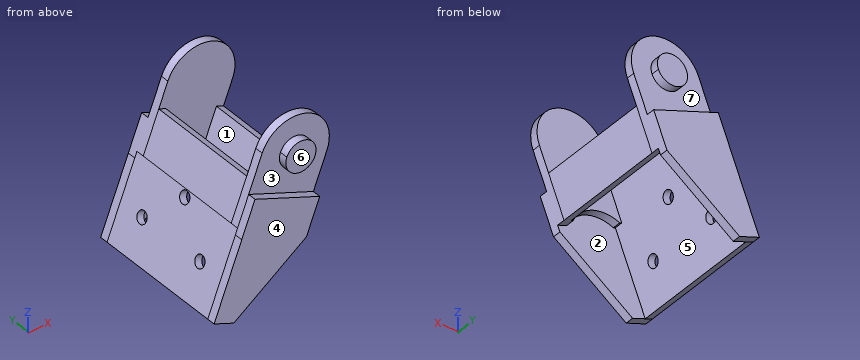
```python
from build123d import *

# Parameters (mm, degrees)
SALIENTE_EXTRUIR1_START   = -2.75
SALIENTE_EXTRUIR1_DEPTH   = 5.5
SALIENTE_EXTRUIR1_2_DEPTH = 2.75
SALIENTE_EXTRUIR2_DEPTH   = 38
SALIENTE_EXTRUIR3_START   = 2.75
SALIENTE_EXTRUIR3_DEPTH   = 2.75
CROQUIS4_W                = 23
CROQUIS4_H                = 43.5
CORTAR_EXTRUIR1_DEPTH     = 8.25
CORTAR_EXTRUIR2_DEPTH     = 2.75
CROQUIS6_W                = 38
CROQUIS6_H                = 22.249999999
CORTAR_EXTRUIR3_DEPTH     = 16.59246817
CROQUIS7_W                = 3.203765914
CROQUIS7_H                = 38
CORTAR_EXTRUIR4_DEPTH     = 8.25
CROQUIS8_W                = 3.203765916
CROQUIS8_H                = 38
CORTAR_EXTRUIR5_DEPTH     = 8.25
CROQUIS9_W                = 14
CROQUIS9_H                = 38
CORTAR_EXTRUIR6_DEPTH     = 0.703765915
CROQUIS10_W               = 14
CROQUIS10_H               = 38
CORTAR_EXTRUIR7_DEPTH     = 0.703765915
SALIENTE_EXTRUIR4_START   = 2.75
SALIENTE_EXTRUIR4_DEPTH   = 2.75
CORTAR_EXTRUIR8_DEPTH     = 2.75
CROQUIS13_W               = 12.249999999
CROQUIS13_H               = 2.75
CORTAR_EXTRUIR9_DEPTH     = 74.034358614
CROQUIS14_W               = 12.249999999
CROQUIS14_H               = 2.75
CORTAR_EXTRUIR10_DEPTH    = 74.034358614
CROQUIS15_W               = 5
CROQUIS15_H               = 2.75
CROQUIS16_W               = 5
CROQUIS16_H               = 2.75
TALADRO1_D                = 10.15
TALADRO1_DEPTH            = 2.75
TALADRO2_D                = 10.15
CORTAR_EXTRUIR11_DEPTH    = 2.75
CORTAR_EXTRUIR12_START    = -2.75
CORTAR_EXTRUIR12_DEPTH    = 2.75
CORTAR_EXTRUIR13_REACH    = 202.135
SALIENTE_EXTRUIR5_DEPTH   = 2.75
SALIENTE_EXTRUIR6_DEPTH   = 2.75
CROQUIS26_W               = 27
CROQUIS26_H               = 43.5
SALIENTE_EXTRUIR7_DEPTH   = 2.5
CROQUIS27_R               = 2
CORTAR_EXTRUIR14_DEPTH    = 2.5


with BuildPart() as part:
    # Saliente-Extruir1: read off the stored shape, not the designer's step
    # Saliente-Extruir1 outline → Saliente-Extruir1 (new body)
    with BuildSketch(Plane(origin=(0, 40.75, 0), x_dir=(-1, 0, 0), z_dir=(0, 1, 0)).offset(SALIENTE_EXTRUIR1_START)):
        with BuildLine():
            Line((161.177139208, 19.345694485), (182.584423689, 27.755698719))
            Line((182.584423689, 27.755698719), (171.432026769, 56.143619441))
            ThreePointArc((171.432026769, 56.143619441), (156.523382412, 62.642259564), (150.024742289, 47.733615207))
            Line((150.024742289, 47.733615207), (161.177139208, 19.345694485))
        make_face()
    extrude(amount=SALIENTE_EXTRUIR1_DEPTH)

    # Saliente-Extruir1 2 outline → Saliente-Extruir1 2 (add)
    with BuildSketch(Plane(origin=(0, 40.75, 0), x_dir=(-1, 0, 0), z_dir=(0, 1, 0))):
        with BuildLine():
            ThreePointArc((161.177139208, 19.345694485), (176.085783565, 12.847054362), (182.584423687, 27.755698719))
            Line((182.584423687, 27.755698719), (161.177139208, 19.345694485))
        make_face()
    extrude(amount=SALIENTE_EXTRUIR1_2_DEPTH)

    # Croquis2 → Saliente-Extruir2 (add)
    with BuildSketch(Plane.XZ.offset(-38)):
        Polygon((-171.432026768, 56.143619442), (-150.024742288, 47.733615205), (-161.177139209, 19.345694483), (-182.584423689, 27.755698719), align=None)
    extrude(amount=SALIENTE_EXTRUIR2_DEPTH)

    # Croquis3 → Saliente-Extruir3 (add)
    with BuildSketch(Plane.XZ.offset(SALIENTE_EXTRUIR3_START)):
        with BuildLine():
            Line((-182.584423688, 27.755698719), (-171.432026768, 56.143619441))
            ThreePointArc((-171.432026768, 56.143619441), (-156.523382412, 62.642259564), (-150.024742289, 47.733615207))
            Line((-150.024742289, 47.733615207), (-161.177139208, 19.345694485))
            Line((-161.177139208, 19.345694485), (-182.584423688, 27.755698719))
        make_face()
    extrude(amount=-SALIENTE_EXTRUIR3_DEPTH)

    # Croquis4 → Cortar-Extruir1 (cut)
    with BuildSketch(Plane(origin=(-14.965700114, 0, -38.094511116), x_dir=(-0.9307514991056489, 0, 0.3656523580022251), z_dir=(-0.3656523580022251, 0, -0.9307514991056489))):
        with Locations((168.589662745, 19)):
            Rectangle(CROQUIS4_W, CROQUIS4_H)
    extrude(amount=-CORTAR_EXTRUIR1_DEPTH, mode=Mode.SUBTRACT)

    # Croquis5 → Cortar-Extruir2 (cut)
    with BuildSketch(Plane(origin=(0, 40.75, 0), x_dir=(1, 0, 0), z_dir=(0, 1, 0))):
        with BuildLine():
            Line((-161.142417183, -28.195858914), (-176.585881806, -34.262934025))
            ThreePointArc((-176.585881806, -34.262934025), (-167.602648859, -34.440489141), (-161.142417183, -28.195858914))
        make_face()
    extrude(amount=-CORTAR_EXTRUIR2_DEPTH, mode=Mode.SUBTRACT)

    # Croquis6 → Cortar-Extruir3 (cut)
    with BuildSketch(Plane(origin=(-149.193349022, 0, 58.611670162), x_dir=(0, 1, 0), z_dir=(0.9307514991056486, 0, -0.3656523580022258))):
        with Locations((19, -21.553766865)):
            Rectangle(CROQUIS6_W, CROQUIS6_H)
    extrude(amount=-CORTAR_EXTRUIR3_DEPTH, mode=Mode.SUBTRACT)

    # Croquis7 → Cortar-Extruir4 (cut)
    with BuildSketch(Plane(origin=(-3.8133032, 0, -9.706590403), x_dir=(0.9307514990825102, 0, -0.36565235806112356), z_dir=(0.36565235806112356, 0, 0.9307514990825102))):
        with Locations((-158.691545702, 19)):
            Rectangle(CROQUIS7_W, CROQUIS7_H)
    extrude(amount=-CORTAR_EXTRUIR4_DEPTH, mode=Mode.SUBTRACT)

    # Croquis8 → Cortar-Extruir5 (cut)
    with BuildSketch(Plane(origin=(-3.8133032, 0, -9.706590403), x_dir=(0.9307514990825102, 0, -0.36565235806112356), z_dir=(0.36565235806112356, 0, 0.9307514990825102))):
        with Locations((-178.487779787, 19)):
            Rectangle(CROQUIS8_W, CROQUIS8_H)
    extrude(amount=-CORTAR_EXTRUIR5_DEPTH, mode=Mode.SUBTRACT)

    # Croquis9 → Cortar-Extruir6 (cut)
    with BuildSketch(Plane(origin=(-164.636813645, 0, 64.678745273), x_dir=(-0.3656523580022247, 0, -0.930751499105649), z_dir=(0.930751499105649, 1.4355340193330324e-15, -0.3656523580022247))):
        with Locations((25.678766864, 19)):
            Rectangle(CROQUIS9_W, CROQUIS9_H)
    extrude(amount=-CORTAR_EXTRUIR6_DEPTH, mode=Mode.SUBTRACT)

    # Croquis10 → Cortar-Extruir7 (cut)
    with BuildSketch(Plane(origin=(-149.193349022, 0, 58.611670162), x_dir=(0.3656523580022248, 0, 0.930751499105649), z_dir=(-0.930751499105649, -1.4355340193330322e-15, 0.3656523580022248))):
        with Locations((-25.678766864, 19)):
            Rectangle(CROQUIS10_W, CROQUIS10_H)
    extrude(amount=-CORTAR_EXTRUIR7_DEPTH, mode=Mode.SUBTRACT)

    # Croquis11 → Saliente-Extruir4 (add)
    with BuildSketch(Plane.XZ.offset(2.75).offset(SALIENTE_EXTRUIR4_START)):
        with BuildLine():
            Line((-150.024742289, 47.733615207), (-161.177139208, 19.345694485))
            ThreePointArc((-161.177139208, 19.345694485), (-176.085783565, 12.847054362), (-182.584423687, 27.755698719))
            Line((-182.584423687, 27.755698719), (-171.432026769, 56.143619441))
            ThreePointArc((-171.432026769, 56.143619441), (-156.523382412, 62.642259564), (-150.024742289, 47.733615207))
        make_face()
    extrude(amount=-SALIENTE_EXTRUIR4_DEPTH)

    # Croquis12 → Cortar-Extruir8 (cut)
    with BuildSketch(Plane(origin=(0, 0, 0), x_dir=(-1, 0, 0), z_dir=(0, 1, 0))):
        with BuildLine():
            Line((161.142417183, 28.195858914), (176.585881806, 34.262934025))
            ThreePointArc((176.585881806, 34.262934025), (167.602648859, 34.440489141), (161.142417183, 28.195858914))
        make_face()
    extrude(amount=-CORTAR_EXTRUIR8_DEPTH, mode=Mode.SUBTRACT)

    # Croquis13 → Cortar-Extruir9 (cut, through all)
    with BuildSketch(Plane(origin=(-146.211439094, 0, 57.440205601), x_dir=(-0.36565235800222584, 0, -0.9307514991056486), z_dir=(0.9307514991056486, 0, -0.36565235800222584))):
        with Locations((16.553766864, -4.125)):
            Rectangle(CROQUIS13_W, CROQUIS13_H)
    extrude(amount=-CORTAR_EXTRUIR9_DEPTH, mode=Mode.SUBTRACT)

    # Croquis14 → Cortar-Extruir10 (cut, through all)
    with BuildSketch(Plane(origin=(-146.211439094, 0, 57.440205601), x_dir=(-0.36565235800222584, 0, -0.9307514991056486), z_dir=(0.9307514991056486, 0, -0.36565235800222584))):
        with Locations((16.553766864, 42.125)):
            Rectangle(CROQUIS14_W, CROQUIS14_H)
    extrude(amount=-CORTAR_EXTRUIR10_DEPTH, mode=Mode.SUBTRACT)

    # Croquis15 → Revolución1 (revolve)
    with BuildSketch(Plane(origin=(0, 0, 51.938617325), x_dir=(-1, 0, 0), z_dir=(0, 0, -1))):
        with Locations((158.228384529, -4.125)):
            Rectangle(CROQUIS15_W, CROQUIS15_H)
    revolve(axis=Axis((-160.728384529, -5.5, 51.938617325), (0, 1, 0)))

    # Croquis16 → Revolución2 (revolve)
    with BuildSketch(Plane(origin=(0, 0, 51.938617325), x_dir=(-1, 0, 0), z_dir=(0, 0, -1))):
        with Locations((158.228384529, 42.125)):
            Rectangle(CROQUIS16_W, CROQUIS16_H)
    revolve(axis=Axis((-160.728384529, 40.75, 51.938617325), (0, 1, 0)))

    # Taladro1
    with Locations(Plane(origin=(0, -5.5, 0), x_dir=(-1, 0, 0), z_dir=(0, -1, 0))):
        with Locations((171.880781448, -23.550696602)):
            Hole(TALADRO1_D / 2, depth=TALADRO1_DEPTH)

    # Taladro2 (through all)
    with Locations(Plane(origin=(0, 40.75, 0), x_dir=(-1, 0, 0), z_dir=(0, -1, 0))):
        with Locations((171.880781448, -23.550696602)):
            Hole(TALADRO2_D / 2)

    # Croquis21 → Cortar-Extruir11 (cut)
    with BuildSketch(Plane.XZ.offset(5.5)):
        with BuildLine():
            ThreePointArc((-165.382142024, 53.766879114), (-158.900122739, 56.59237482), (-156.074627033, 50.110355534))
            Line((-156.074627033, 50.110355534), (-150.024742289, 47.733615207))
            ThreePointArc((-150.024742289, 47.733615207), (-156.523382412, 62.642259564), (-171.432026769, 56.143619441))
            Line((-171.432026769, 56.143619441), (-165.382142024, 53.766879114))
        make_face()
    extrude(amount=-CORTAR_EXTRUIR11_DEPTH, mode=Mode.SUBTRACT)

    # Croquis22 → Cortar-Extruir12 (cut)
    with BuildSketch(Plane(origin=(0, 43.5, 0), x_dir=(1, 0, 0), z_dir=(0, 1, 0)).offset(CORTAR_EXTRUIR12_START)):
        with BuildLine():
            ThreePointArc((-165.382142024, -53.766879115), (-158.900122739, -56.59237482), (-156.074627033, -50.110355534))
            Line((-156.074627033, -50.110355534), (-150.024742289, -47.733615207))
            ThreePointArc((-150.024742289, -47.733615207), (-156.523382412, -62.642259564), (-171.432026769, -56.143619442))
            Line((-171.432026769, -56.143619442), (-165.382142024, -53.766879115))
        make_face()
    extrude(amount=CORTAR_EXTRUIR12_DEPTH, mode=Mode.SUBTRACT)

    # Cortar-Extruir13: up to this face of the body (flat: up to its plane)
    cortar_extruir13_end = Plane(part.part.faces().sort_by_distance((-169.996704911, 43.5, 28.346528005))[0])
    # Croquis23 → Cortar-Extruir13 (cut, up to the picked face)
    with BuildSketch(Plane.XZ.offset(5.5), mode=Mode.PRIVATE) as cortar_extruir13_sk1:
        Polygon((-180.29909645, 33.572895588), (-158.891811971, 25.162891354), (-166.204859131, 6.547861372), (-187.61214361, 14.957865606), align=None)
    cortar_extruir13_tool1 = split(extrude(cortar_extruir13_sk1.sketch, amount=-CORTAR_EXTRUIR13_REACH, mode=Mode.PRIVATE), bisect_by=cortar_extruir13_end, keep=Keep.BOTH, mode=Mode.PRIVATE)
    add(cortar_extruir13_tool1.solids().sort_by(Axis((-173.251978, -5.5, 20.060378), (0, 1, 0)))[0], mode=Mode.SUBTRACT)

    # Croquis24 → Saliente-Extruir5 (add)
    with BuildSketch(Plane.XZ.offset(5.5)):
        Polygon((-180.29909645, 33.572895588), (-189.4404054, 10.304108111), (-182.925144906, 7.744541605), (-158.891811971, 25.162891354), align=None)
    extrude(amount=-SALIENTE_EXTRUIR5_DEPTH)

    # Croquis25 → Saliente-Extruir6 (add)
    with BuildSketch(Plane(origin=(0, 43.5, 0), x_dir=(1, 0, 0), z_dir=(0, 1, 0))):
        Polygon((-180.29909645, -33.572895588), (-189.4404054, -10.304108111), (-182.925144906, -7.744541605), (-158.891811971, -25.162891354), align=None)
    extrude(amount=-SALIENTE_EXTRUIR6_DEPTH)

    # Croquis26 → Saliente-Extruir7 (add)
    with BuildSketch(Plane(origin=(-167.618723573, 0, 65.850209835), x_dir=(0.36565235800222584, 0, 0.9307514991056486), z_dir=(-0.9307514991056486, 0, 0.36565235800222584))):
        with Locations((-46.178766864, 19)):
            Rectangle(CROQUIS26_W, CROQUIS26_H)
    extrude(amount=-SALIENTE_EXTRUIR7_DEPTH)

    # Croquis27 → Cortar-Extruir14 (cut)
    with BuildSketch(Plane(origin=(-167.618723573, 0, 65.850209835), x_dir=(0.36565235800222584, 0, 0.9307514991056486), z_dir=(-0.9307514991056486, 0, 0.36565235800222584))):
        with Locations((-47.428766864, 31.5)):
            Circle(CROQUIS27_R)
        with Locations((-47.428766864, 6.5)):
            Circle(CROQUIS27_R)
        with Locations((-34.928766864, 19)):
            Circle(CROQUIS27_R)
    extrude(amount=-CORTAR_EXTRUIR14_DEPTH, mode=Mode.SUBTRACT)


solid = part.part
```
Work out the finished part from the listing and answer in its coordinate system (mm). Face numbers are marked on the shaded views. A direction names the side the tool comes from. Coordinates: 2 decimals unless noted, no trailing zeros. Order: outer loops, then holes, each group sorted by start corner. A loop starts at its lowest first (then second) coordinate and runs counter-clockwise, first axis right, second up. Notation, with made-up numbers: (32, 74.25) - (67, 74.25) arc R22 cw to (67, 110.25) - close; hole circle Ø8 at (4, -26). An arc over 180 degrees is marked (long way). Answer as a JSON object with one key per item and string values.
1. Find section D-D on z = 38.5. Determine the outline of the cut face in (x, y), plus the area to 3 significant figures.
Output values:
{"outline": "(-178.36, -5.5) - (-160.02, -5.5) - (-160.02, -2.75) - (-153.65, -2.75) - (-153.65, 40.75) - (-160.02, 40.75) - (-160.02, 43.5) - (-178.36, 43.5) - close; hole (-175.68, 0) - (-156.34, 0) - (-156.34, 38) - (-175.68, 38) - close", "area": "441 mm²"}
2. Find section C-C on x = -162. Determine the outline of the cut face in (y, z).
Output values:
{"outline": "(-5.5, 22.91) - (-2.75, 22.91) - (-2.75, 29.82) - (0, 29.82) - (0, 63.37) - (-2.75, 63.37) - (-2.75, 56.77) - (-5.5, 56.77) - (-5.5, 47.1) - (-2.75, 47.1) - (-2.75, 39.28) - (-5.5, 39.28) - close; (38, 29.82) - (40.75, 29.82) - (40.75, 22.91) - (43.5, 22.91) - (43.5, 39.28) - (40.75, 39.28) - (40.75, 47.1) - (43.5, 47.1) - (43.5, 56.77) - (40.75, 56.77) - (40.75, 63.37) - (38, 63.37) - close"}
3. A tool of negligible diameter and unlimited length cuts with its end or side. For the marked faces 1, 2, 3 and 4, from which of +Z, -Z, +X, -X, +Y, -Y can it reach the whole face along a straight path? Write none if from no direction.
Output values:
{"face 1": "+Z", "face 2": "-Z", "face 3": "-Y", "face 4": "+Z, -Z, +X, -X, -Y"}
4. Each of these flat-tipped pins is pushed along its axis until it touches: P1, Ø1, axis at y = 21.5, z = 45.5, coming from the +X side; P2, Ø1.5, axis at y = 24.5, z = 13.5, coming from the +X side; P3, Ø6, axis at y = 33.5, z = 40.5, coming from the -X side. Where does it stop, or does it pass through?
Output values:
{"P1": "stops at x = -172.73", "P2": "stops at x = -185.2", "P3": "stops at x = -178.76"}
5. Find section A-A on y = 15.5. Determine the outline of the cut face in (x, z), plus the area to 4 significant figures.
Output values:
{"outline": "(-189.44, 10.3) - (-187.11, 9.39) - (-172.12, 47.55) - (-174.45, 48.46) - close; (-160.49, 27.94) - (-158.16, 27.02) - (-153.04, 40.05) - (-155.37, 40.97) - close", "area": "137.5 mm²"}
6. The mould has two halves that part along Y. Classify the marked faces 5, 6 and 7: +Y half, -Y half, draft (parallel to the pull), parting line (faces both ways), or undercut.
Output values:
{"face 5": "undercut", "face 6": "-Y half", "face 7": "+Y half"}
7. Find section B-B on y = 39. Determine the outline of the cut face in (x, z), plus the area to 3 significant figures.
Output values:
{"outline": "(-189.44, 10.3) - (-187.11, 9.39) - (-177.24, 34.52) - (-176.59, 34.26) arc R11.7 cw to (-161.14, 28.2) - (-158.16, 27.02) - (-150.02, 47.73) arc R11.5 ccw to (-171.43, 56.14) - close", "area": "748 mm²"}
8. Consider line 1 (Y direction, x = -168.5, z = 31); line 2 (Y direction, x = -157, z = 50.5); line 3 (X direction, y = 35.5, z = 16.5). Determine where each line is inside the solid, lowest interval first.
Output values:
{"line 1": "y = -5.5 to -2.75, 40.75 to 43.5", "line 2": "y = -5.5 to 0, 38 to 43.5", "line 3": "x = -187.01 to -184.32"}
